Model file for the job. Use its own axes, mm. Round coordinates to 2 decimals unless told otherwise and drop trailing zeros. Order: outer loops, then holes, each group sorted by start corner. A loop starts at its lowest first (then second) coordinate and runs counter-clockwise, first axis right, second up. Notation, with made-up numbers: (7.5, 10) -> (29.5, 10) arc R27 cw to (29.5, 48) -> close; hole circle Ø4 at (-18.75, 79.25). An arc over 180 degrees is marked (long way). Answer as CSV lines item,"result".
```python
from build123d import *

# Parameters (mm, degrees)
SKETCH1_W           = 150
SKETCH1_H           = 195
SKETCH1_W_2         = 60
SKETCH1_H_2         = 30
BOSS_EXTRUDE1_DEPTH = 1
SKETCH2_R           = 6
CUT_EXTRUDE1_DEPTH  = 2


with BuildPart() as part:
    # Sketch1 → Boss-Extrude1 (new body)
    with BuildSketch(Plane.XY):
        with Locations((80.10402455, 77.161264357)):
            Rectangle(SKETCH1_W, SKETCH1_H)
        with Locations((42.10402455, 149.661264357)):
            Rectangle(SKETCH1_W_2, SKETCH1_H_2, mode=Mode.SUBTRACT)
        with Locations((122.10402455, 149.661264357)):
            Rectangle(SKETCH1_W_2, SKETCH1_H_2, mode=Mode.SUBTRACT)
        with Locations((42.10402455, 4.661264357)):
            Rectangle(SKETCH1_W_2, SKETCH1_H_2, mode=Mode.SUBTRACT)
        with Locations((122.10402455, 4.661264357)):
            Rectangle(SKETCH1_W_2, SKETCH1_H_2, mode=Mode.SUBTRACT)
    extrude(amount=BOSS_EXTRUDE1_DEPTH)

    # Sketch2 → Cut-Extrude1 (cut)
    with BuildSketch(Plane.XY.offset(1)):
        with Locations((25.10402455, 119.661264357)):
            Circle(SKETCH2_R)
        with Locations((25.10402455, 94.661264357)):
            Circle(SKETCH2_R)
        with Locations((25.10402455, 69.661264357)):
            Circle(SKETCH2_R)
        with Locations((25.10402455, 44.661264357)):
            Circle(SKETCH2_R)
        with Locations((52.60402455, 119.661264357)):
            Circle(SKETCH2_R)
        with Locations((52.60402455, 69.661264357)):
            Circle(SKETCH2_R)
        with Locations((52.60402455, 94.661264357)):
            Circle(SKETCH2_R)
        with Locations((52.60402455, 44.661264357)):
            Circle(SKETCH2_R)
        with Locations((80.10402455, 119.661264357)):
            Circle(SKETCH2_R)
        with Locations((80.10402455, 69.661264357)):
            Circle(SKETCH2_R)
        with Locations((80.10402455, 94.661264357)):
            Circle(SKETCH2_R)
        with Locations((80.10402455, 44.661264357)):
            Circle(SKETCH2_R)
        with Locations((107.60402455, 119.661264357)):
            Circle(SKETCH2_R)
        with Locations((107.60402455, 69.661264357)):
            Circle(SKETCH2_R)
        with Locations((107.60402455, 94.661264357)):
            Circle(SKETCH2_R)
        with Locations((107.60402455, 44.661264357)):
            Circle(SKETCH2_R)
        with Locations((135.10402455, 119.661264357)):
            Circle(SKETCH2_R)
        with Locations((135.10402455, 69.661264357)):
            Circle(SKETCH2_R)
        with Locations((135.10402455, 94.661264357)):
            Circle(SKETCH2_R)
        with Locations((135.10402455, 44.661264357)):
            Circle(SKETCH2_R)
    extrude(amount=-CUT_EXTRUDE1_DEPTH, mode=Mode.SUBTRACT)


solid = part.part
```
Q1. Mould opens along Y. For faces 1 (the cylindrical face through (48.182, 73.716, 0.507)), 2 (the flat face through (79, 79, 0)) say: +Y half, -Y half, draft (parallel to the pull), parting line (faces both ways), or undercut.
Checks:
face 1,"undercut"
face 2,"draft"
Q2. Flat gauge pin, fed straight in: pin 1 (15.5 mm diameter, centred on x = 25.1, y = 119.66, fed in from -Z). Where does the tip first touch, or does it go through?
Checks:
pin 1,"z = 0"
Q3. Wall check: L1, parallel to Y at x = 118.5, z = 0.35; L2, parallel to X at y = 10, z = 0.75; L3, parallel to X at y = 72.5, z = 0.7. Give the ranges that are in metal, low to high. Write a range as [from, to].
Checks:
L1,"[-20.34, -10.34], [19.66, 134.66], [164.66, 174.66]"
L2,"[5.1, 12.1], [72.1, 92.1], [152.1, 155.1]"
L3,"[5.1, 19.82], [30.39, 47.32], [57.89, 74.82], [85.39, 102.32], [112.89, 129.82], [140.39, 155.1]"
Q4. Saw through at C-C (x = 81). Write the cut outline in (y, z), plus the area to 3 significant figures.
Checks:
outline,"(-20.34, 0) -> (38.73, 0) -> (38.73, 1) -> (-20.34, 1) -> close; (50.59, 0) -> (63.73, 0) -> (63.73, 1) -> (50.59, 1) -> close; (75.59, 0) -> (88.73, 0) -> (88.73, 1) -> (75.59, 1) -> close; (100.59, 0) -> (113.73, 0) -> (113.73, 1) -> (100.59, 1) -> close; (125.59, 0) -> (174.66, 0) -> (174.66, 1) -> (125.59, 1) -> close"
area,"148 mm²"
Q5. Saw through at D-D (y = 42). Write the cut outline in (x, z).
Checks:
outline,"(5.1, 0) -> (19.73, 0) -> (19.73, 1) -> (5.1, 1) -> close; (30.48, 0) -> (47.23, 0) -> (47.23, 1) -> (30.48, 1) -> close; (57.98, 0) -> (74.73, 0) -> (74.73, 1) -> (57.98, 1) -> close; (85.48, 0) -> (102.23, 0) -> (102.23, 1) -> (85.48, 1) -> close; (112.98, 0) -> (129.73, 0) -> (129.73, 1) -> (112.98, 1) -> close; (140.48, 0) -> (155.1, 0) -> (155.1, 1) -> (140.48, 1) -> close"
Q6. Saw through at A-A (y = 149). Write the cut outline in (x, z), plus the area to 3 significant figures.
Checks:
outline,"(5.1, 0) -> (12.1, 0) -> (12.1, 1) -> (5.1, 1) -> close; (72.1, 0) -> (92.1, 0) -> (92.1, 1) -> (72.1, 1) -> close; (152.1, 0) -> (155.1, 0) -> (155.1, 1) -> (152.1, 1) -> close"
area,"30.0 mm²"
Q7. Saw through at B-B (x = 120.5). Write the cut outline in (y, z), plus the area to 3 significant figures.
Checks:
outline,"(-20.34, 0) -> (-10.34, 0) -> (-10.34, 1) -> (-20.34, 1) -> close; (19.66, 0) -> (134.66, 0) -> (134.66, 1) -> (19.66, 1) -> close; (164.66, 0) -> (174.66, 0) -> (174.66, 1) -> (164.66, 1) -> close"
area,"135 mm²"
